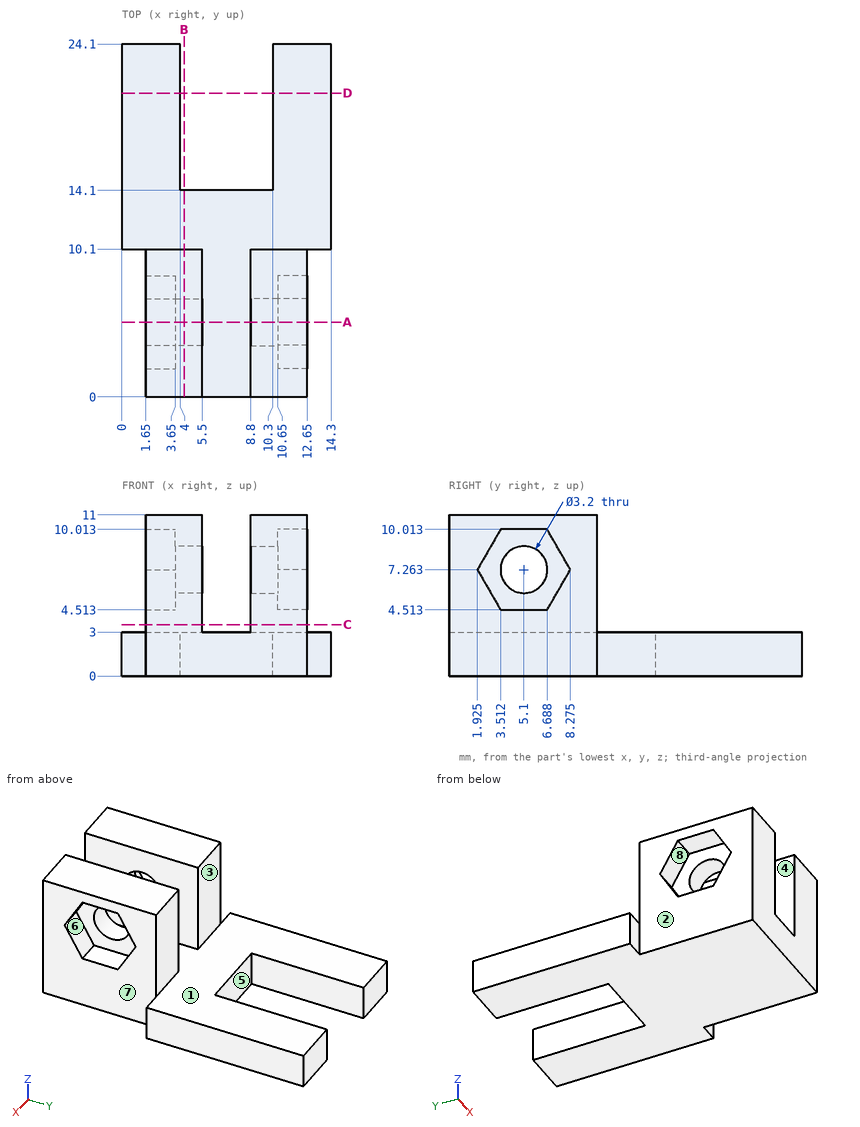
Job drawing, mm, ordinate dimensions from the low corner. One solid piece. A direction names the side the tool comes from. Coordinates: 2 decimals unless noted, no trailing zeros. Write each loop counter-clockwise with the first axis right and the second up, starting at its lowest first coordinate (ties: lowest second). Pieces come first, ordered by that corner, then holes.
Item 1: Slice it at D-D (y = 20.75). Write the cut outline in (x, z).
Item 2: Slice it at A-A (y = 5.1). Write the cut outline in (x, z).
Item 3: Which spindle directions (+Z, -Z, +X, -X, +Y, -Y) get a long thin tool onto all of the face, cutting with end or side? Do the marked faces 5, 6, 7 and 8. Say none if no direction does.
Item 4: Slice it at C-C (z = 3.5). Write the cut outline in (x, y).
Item 5: Probe line 1 (X direction, y = 2.75, z = 3.75); line 2 (Z direction, x = 4.85, y = 5.1); line 3 (Y direction, x = 4.75, z = 0.75). List the from-to ranges inside material, lowest first.
Item 6: Slice it at B-B (x = 4.25). Write the cut outline in (y, z).
Item 7: Pin check, flat tips, straight feed: pin 1 (2.5 mm diameter, centred on y = 2.5, z = 8, fed in from -X); pin 2 (1.5 mm diameter, centred on x = 12.5, y = 19, fed in from +Z); pin 3 (1.3 mm diameter, centred on x = 13.5, z = 2, fed in from -Y); pin 4 (2.5 mm diameter, centred on y = 5.1, z = 7.26, fed in from -X). Stop position of each tip, or through.
Item 8: Mould opens along X. For the marked faces 1, 2, 3 and 4 say: released by +X, released by -X, zero draft, split by the parting line, or undercut.
Results found:
1. outline: (0, 0) - (4, 0) - (4, 3) - (0, 3) - close; (10.3, 0) - (14.3, 0) - (14.3, 3) - (10.3, 3) - close
2. outline: (1.65, 0) - (12.65, 0) - (12.65, 4.51) - (10.65, 4.51) - (10.65, 5.66) - (8.8, 5.66) - (8.8, 3) - (5.5, 3) - (5.5, 5.66) - (3.65, 5.66) - (3.65, 4.51) - (1.65, 4.51) - close; (1.65, 10.01) - (3.65, 10.01) - (3.65, 8.86) - (5.5, 8.86) - (5.5, 11) - (1.65, 11) - close; (8.8, 8.86) - (10.65, 8.86) - (10.65, 10.01) - (12.65, 10.01) - (12.65, 11) - (8.8, 11) - close
3. face 5: +Z, -Z, +Y
3. face 6: +X
3. face 7: +Z, -Z, +X, -Y
3. face 8: -X
4. outline: (1.65, 0) - (5.5, 0) - (5.5, 10.1) - (1.65, 10.1) - close; (8.8, 0) - (12.65, 0) - (12.65, 10.1) - (8.8, 10.1) - close
5. line 1: x = 1.65 to 5.5, 8.8 to 12.65
5. line 2: z = 0 to 5.66, 8.86 to 11
5. line 3: y = 0 to 14.1
6. outline: (0, 0) - (14.1, 0) - (14.1, 3) - (10.1, 3) - (10.1, 11) - (0, 11) - close; hole circle Ø3.2 at (5.1, 7.26)
7. pin 1: stops at x = 1.65
7. pin 2: stops at z = 3
7. pin 3: stops at y = 10.1
7. pin 4: passes through
8. face 1: undercut
8. face 2: released by -X
8. face 3: zero draft
8. face 4: undercut
